Check sheet for the modelled part. Datum: model origin and axes. Units: mm. A direction names the side the tool comes from. Round coordinates to 2 decimals unless told otherwise and drop trailing zeros. Loops run counter-clockwise (first coordinate to the right, second up) from the corner with the lowest first, then second, coordinate; pieces in that order, holes last. Notation, with made-up numbers: M 29.25,31.5 L 77.25,31.5 A18 cw 77.25,40.5 Z; hole C 47.5,-32.5 d6. An arc over 180 degrees is marked long. One line per question, with ' | ' between items. Start each with the question number.
(1) Section check D-D (y = -30). Record the boundary of the cut face in (x, z) (3 decimals), and give its area (3 significant figures).
(2) Section check C-C (x = 28). Record the boundary of the cut face in (y, z) (3 decimals), and give its area (3 significant figures).
(3) Draft check along Y on faces 1 (the face through (-27.715, -21.251, 1.565)), 2 (the face through (0.295, 22.223, 3.131)), 3 (the face through (0, -23, 0)). Enter one of: +Y half, -Y half, draft (parallel to the pull), parting line (faces both ways), or undercut.
(4) Go/stop test with flat-tipped pins: P1, Ø1, axis at x = -20, z = 2.5, coming from the +Y side; P2, Ø3.5, axis at x = 20.5, z = 3.5, coming from the -Y side; P3, Ø3.5, axis at x = -20, z = 4, coming from the -Y side. Record where each tip stops, or that it passes through.
(5) Tool access check on faces 4 (the face through (22.224, -0.189, 3.836)), 5 (the face through (-5.506, -24.796, 4.74)), 6 (the face through (-0.1, -22.5, 6.35)), 7 (the face through (19, 12.954, 3)). Record the directions out of +Z, -Z, +X, -X, +Y, -Y that give a thin tool (end or side, any length) a straight path to the whole face; none if there is none.
(6) Section check A-A (y = 0). Record the boundary of the cut face in (x, z) (3 decimals).
(7) Thickness scan on probe 1 along X at (y, z) = (2, 3); probe 2 along Z at (x, y) = (23.5, -18) (3 decimals); probe 3 along X at (y, z) = (11, 4.5). Record the ranges inside material, lowest first. Write a range as [from, to].
```python
from build123d import *

# Parameters (mm, degrees)
F0_R          = 34.925
F0_R_2        = 25.4
F1_DEPTH      = 3.175
F0_R_3        = 22.225
F2_DEPTH      = 6.35
F3_R          = 22.225
F4_DEPTH      = 12.954
F4_DEPTH_BACK = 12.954


with BuildPart() as f1:
    # F0 (on Top) → F1 (new body)
    with BuildSketch(Plane.XY):
        Circle(F0_R)
        Circle(F0_R_2, mode=Mode.SUBTRACT)
    extrude(amount=F1_DEPTH)

    # F0 (on Top) → F2 (join)
    with BuildSketch(Plane.XY):
        Circle(F0_R_2)
        Circle(F0_R_3, mode=Mode.SUBTRACT)
    extrude(amount=F2_DEPTH)

    # F3 (on Front) → F4 (cut, two sides)
    with BuildSketch(Plane.XZ) as f4_sk:
        with Locations((0, -6.35)):
            Circle(F3_R)
    extrude(amount=-F4_DEPTH, mode=Mode.SUBTRACT)
    extrude(f4_sk.sketch, amount=F4_DEPTH_BACK, mode=Mode.SUBTRACT)


solid = f1.part
```
The answers:
1) outline: M -17.882,0 L 17.882,0 L 17.882,3.175 L -17.882,3.175 Z | area: 114 mm²
2) outline: M -20.875,0 L 20.875,0 L 20.875,3.175 L -20.875,3.175 Z | area: 133 mm²
3) face 1: parting line | face 2: undercut | face 3: draft
4) P1: y = 28.97 | P2: y = -29.45 | P3: y = -29.65
5) face 4: +Z, -Z | face 5: +Z | face 6: +Z, +X, -X, +Y, -Y | face 7: -Z
6) outline: M -34.925,0 L -22.225,0 L -22.225,6.35 L -25.4,6.35 L -25.4,3.175 L -34.925,3.175 Z; M 22.225,0 L 34.925,0 L 34.925,3.175 L 25.4,3.175 L 25.4,6.35 L 22.225,6.35 Z
7) probe 1: [-34.87, -22.13], [22.13, 34.87] | probe 2: [0, 3.175] | probe 3: [-22.89, -19.4], [19.4, 22.89]
